from build123d import *

# Parameters (mm, degrees)
SKETCH_1_W             = 22
SKETCH_1_H             = 13
EXTRUDE_1_DEPTH        = 7.5
SKETCH_2_W             = 6.5
SKETCH_2_H             = 13
EXTRUDE_2_DEPTH        = 1
FILLET_1_R             = 1
SKETCH_3_W             = 2
SKETCH_3_H             = 5.5
EXTRUDE_3_DEPTH        = 0.5
FILLET_2_R             = 1
FILLET_2_OF_MIRROR_1_R = 1
SKETCH_4_W             = 7
SKETCH_4_H             = 5.5
EXTRUDE_4_DEPTH        = 8.6
FILLET_3_R             = 3


with BuildPart() as part:
    # Эскиз1 → Бобышка-Вытянуть1 (new body)
    with BuildSketch(Plane.XY):
        with Locations((11, 6.5)):
            Rectangle(SKETCH_1_W, SKETCH_1_H)
    extrude(amount=EXTRUDE_1_DEPTH)

    # Эскиз2 → Бобышка-Вытянуть2 (add)
    with BuildSketch(Plane.XY.offset(7.5)):
        with Locations((-3.25, 6.5)):
            Rectangle(SKETCH_2_W, SKETCH_2_H)
        with Locations((25.25, 6.5)):
            Rectangle(SKETCH_2_W, SKETCH_2_H)
    extrude(amount=-EXTRUDE_2_DEPTH)

    # Скругление1
    fillet_1_edges = [part.edges().sort_by_distance(p)[0] for p in [
        (28.5, 13, 7),
        (28.5, 0, 7),
        (-6.5, 13, 7),
        (-6.5, 0, 7),
    ]]
    fillet(fillet_1_edges, radius=FILLET_1_R)

    # Эскиз3 → Бобышка-Вытянуть3 (add, symmetric)
    with BuildSketch(Plane(origin=(0, 3.5, 0), x_dir=(-1, 0, 0), z_dir=(0, -1, 0))):
        with Locations((-4, 2.75)):
            Rectangle(SKETCH_3_W, SKETCH_3_H)
        with Locations((-18, 2.75)):
            Rectangle(SKETCH_3_W, SKETCH_3_H)
        with Locations((-11, 2.75)):
            Rectangle(SKETCH_3_W, SKETCH_3_H)
    extrude_3 = extrude(amount=EXTRUDE_3_DEPTH, both=True)

    # Скругление2
    fillet_2_edges = [part.edges().sort_by_distance(p)[0] for p in [
        (19, 3.5, -5.5),
        (17, 3.5, -5.5),
        (12, 3.5, -5.5),
        (10, 3.5, -5.5),
        (5, 3.5, -5.5),
        (3, 3.5, -5.5),
    ]]
    fillet(fillet_2_edges, radius=FILLET_2_R - 0.0001)  # a hair under: the kernel refuses the full size

    # Зеркальное отражение1: Бобышка-Вытянуть3 across plane
    add(extrude_3.mirror(Plane(origin=(0, 6.5, 0), x_dir=(0, 0, 1), z_dir=(0, -1, 0))))

    # Скругление2 of Зеркальное отражение1
    fillet_2_of_mirror_1_edges = [part.edges().sort_by_distance(p)[0] for p in [
        (19, 9.5, -5.5),
        (17, 9.5, -5.5),
        (12, 9.5, -5.5),
        (10, 9.5, -5.5),
        (5, 9.5, -5.5),
        (3, 9.5, -5.5),
    ]]
    fillet(fillet_2_of_mirror_1_edges, radius=FILLET_2_OF_MIRROR_1_R - 0.0001)  # a hair under: the kernel refuses the full size

    # Эскиз4 → Бобышка-Вытянуть4 (add)
    with BuildSketch(Plane.XY.offset(7.5)):
        with Locations((8, 6.5)):
            Rectangle(SKETCH_4_W, SKETCH_4_H)
    extrude_4 = extrude(amount=EXTRUDE_4_DEPTH)

    # Скругление3
    fillet_3_edges = [part.edges().sort_by_distance(p)[0] for p in [
        (11.5, 6.5, 16.1),
        (4.5, 6.5, 16.1),
    ]]
    fillet(fillet_3_edges, radius=FILLET_3_R)

    # Зеркальное отражение4: Бобышка-Вытянуть4 across plane
    add(extrude_4.mirror(Plane(origin=(11, 0, 0), x_dir=(0, 0, 1), z_dir=(1, 0, 0))))


solid = part.part
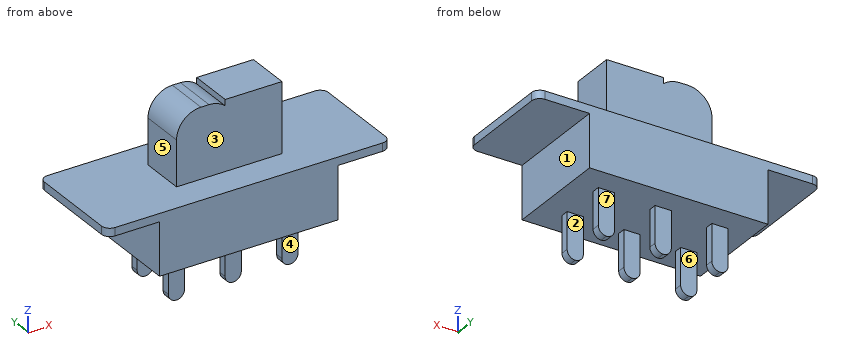
Geometry check sheet. Reference: the model listing, model coordinates, mm. Face numbers are marked on the shaded views. A direction names the side the tool comes from. Coordinates: 2 decimals unless noted, no trailing zeros. Order: outer loops, then holes, each group sorted by start corner. A loop starts at its lowest first (then second) coordinate and runs counter-clockwise, first axis right, second up. Notation, with made-up numbers: (67.5, 78) - (90.5, 78) arc R25 cw to (90.5, 106) - close; hole circle Ø1 at (-32.75, -5). An arc over 180 degrees is marked (long way). One line per item, written item: value.
(1) Sectioned sample at D-D (x = 16.5). Enter the section's corners in (y, z), and give its area (3 significant figures).
Data:
outline: (0, 0) - (13, 0) - (13, 7.5) - (9.25, 7.5) - (9.25, 16.1) - (3.75, 16.1) - (3.75, 7.5) - (0, 7.5) - close
area: 145 mm^2
(2) Sectioned sample at B-B (x = 5.5). Enter the section's corners in (y, z), and give its area (3 significant figures).
Data:
outline: (0, 0) - (13, 0) - (13, 7.5) - (9.25, 7.5) - (9.25, 15.34) - (3.75, 15.34) - (3.75, 7.5) - (0, 7.5) - close
area: 141 mm^2
(3) Thickness scan on probe 1 along Z at (x, y) = (20.5, 10); probe 2 along X at (y, z) = (11.25, 5); probe 3 along X at (y, z) = (8.25, 8.75). Record the ranges inside material, lowest first. Write a range as from..to.
Data:
probe 1: z = 0..7.5
probe 2: x = 0..22
probe 3: x = 4.5..17.5
(4) Access from +Z, -Z, +X, -X, +Y, -Y to the whole of each face (thin tool, end or side, straight path). Record for the marked faces 1, 2, 3 and 4.
Data:
face 1: -Z, +X, +Y, -Y
face 2: -Z, +X, -X
face 3: +Z, +X, -X, -Y
face 4: -Z, +X, -X, -Y
(5) Sectioned sample at C-C (y = 5.25). Enter the section's corners in (x, z).
Data:
outline: (-6.5, 6.5) - (0, 6.5) - (0, 0) - (22, 0) - (22, 6.5) - (28.5, 6.5) - (28.5, 7.5) - (17.5, 7.5) - (17.5, 16.1) - (10.5, 16.1) - (10.5, 15.34) arc R3 ccw to (8.5, 16.1) - (7.5, 16.1) arc R3 ccw to (4.5, 13.1) - (4.5, 7.5) - (-6.5, 7.5) - close
(6) Release check for a two-part mould opening along Y. For the marked faces 5, 6 and 7 record: +Y half, -Y half, draft (parallel to the pull), parting line (faces both ways), or undercut.
Data:
face 5: draft
face 6: undercut
face 7: +Y half
(7) Sectioned sample at A-A (z = -2.5). Enter the section's corners in (x, y).
Data:
outline: (3, 3) - (5, 3) - (5, 4) - (3, 4) - close; (3, 9) - (5, 9) - (5, 10) - (3, 10) - close; (10, 3) - (12, 3) - (12, 4) - (10, 4) - close; (10, 9) - (12, 9) - (12, 10) - (10, 10) - close; (17, 3) - (19, 3) - (19, 4) - (17, 4) - close; (17, 9) - (19, 9) - (19, 10) - (17, 10) - close
(8) Depth check by flat-ended pin: pin 1 Ø6 at (x, y) = (-1.5, 7.5) entering from +Z; pin 2 Ø1 at (x, z) = (17.5, -4) entering from -Y; pin 3 Ø6 at (x, z) = (15.5, 2.5) entering from -Y; pin 4 Ø1 at (x, z) = (18, -3.5) entering from +Y. Enter the tip coordinate at first touch or a pass-through.
Data:
pin 1: stops at z = 7.5
pin 2: stops at y = 3
pin 3: stops at y = 0
pin 4: stops at y = 10
